from build123d import *

# Parameters (mm, degrees)
SKETCH1_W           = 4.7625
SKETCH1_H           = 101.6
BOSS_EXTRUDE1_DEPTH = 34.925
SKETCH2_W           = 101.6
SKETCH2_H           = 3.175
BOSS_EXTRUDE2_DEPTH = 152.4
SKETCH2_4_W         = 1.5875
SKETCH2_4_H         = 3.175
BOSS_EXTRUDE3_DEPTH = 25.4


with BuildPart() as part:
    # Sketch1 → Boss-Extrude1 (new body)
    with BuildSketch(Plane(origin=(0, -30.757642186, 0), x_dir=(-1, 0, 0), z_dir=(0, -1, 0))):
        with Locations((-83.04427371, -7.755970668)):
            Rectangle(SKETCH1_W, SKETCH1_H)
    extrude(amount=-BOSS_EXTRUDE1_DEPTH)

    # Sketch2 → Boss-Extrude2 (add)
    with BuildSketch(Plane.ZY.offset(-80.66302371)):
        with Locations((7.755970668, 2.579857814)):
            Rectangle(SKETCH2_W, SKETCH2_H)
    extrude(amount=BOSS_EXTRUDE2_DEPTH)

    # Sketch2<4> → Boss-Extrude3 (add)
    with BuildSketch(Plane.ZY.offset(-80.66302371)):
        with Locations((-39.075279332, -5.357642186)):
            Rectangle(SKETCH2_4_W, SKETCH2_4_H)
        with Locations((54.587220668, -5.357642186)):
            Rectangle(SKETCH2_4_W, SKETCH2_4_H)
    extrude(amount=BOSS_EXTRUDE3_DEPTH)


solid = part.part
Geometry: final body of the model. Coordinates: model frame, mm. A direction names the side the tool comes from. Coordinates: 2 decimals unless noted, no trailing zeros. Order: outer loops, then holes, each group sorted by start corner. A loop starts at its lowest first (then second) coordinate and runs counter-clockwise, first axis right, second up.
1) Set-up query: faces 4 (the flat face through (68, -5, -39.869)), 5 (the flat face through (68, -5, 53.793)), 6 (the flat face through (-71.737, 3, 7)), 7 (the flat face through (68, -5, 55.381)). Return all of +Z, -Z, +X, -X, +Y, -Y with unobstructed straight access to the full face (end or side cutting, diameter ignored); none if empty.
Result sheet:
face 4: -Z, -X, -Y
face 5: -X, -Y
face 6: +Z, -Z, -X, +Y, -Y
face 7: +Z, -X, -Y
2) Section C-C (y = -9). Return loops of the section in (x, z), then the cut area to 3 significant figures.
Result sheet:
outline: (80.66, -43.04) - (85.43, -43.04) - (85.43, 58.56) - (80.66, 58.56) - close
area: 484 mm2
3) Section D-D (x = 44). Return loops of the section in (y, z).
Result sheet:
outline: (0.99, -43.04) - (4.17, -43.04) - (4.17, 58.56) - (0.99, 58.56) - close
4) Draft query along Z for faces 1 (the flat face through (68, -5, -38.282)), 2 (the flat face through (6, 0.992, 7)), 3 (the flat face through (30, 2, 58.556)). Return one class per face: released by +Z, released by -Z, zero draft, split by the parting line, or undercut.
Result sheet:
face 1: undercut
face 2: zero draft
face 3: released by +Z
5) Section B-B (z = 30.5). Return loops of the section in (x, y), then the cut area to 3 significant figures.
Result sheet:
outline: (-71.74, 0.99) - (80.66, 0.99) - (80.66, -30.76) - (85.43, -30.76) - (85.43, 4.17) - (-71.74, 4.17) - close
area: 650 mm2
6) First-contact query: P1, Ø8, axis at y = -10.5, z = -12.5, coming from the -X side; P2, Ø3.5, axis at x = 70, y = -6, coming from the +Z side; P3, Ø8, axis at x = 36, z = -8, coming from the -Y side. Flat tips, straight axial feed; report the tip coordinate or a pass-through.
Result sheet:
P1: stops at x = 80.66
P2: stops at z = 55.38
P3: stops at y = 0.99
7) Section A-A (x = 74). Return loops of the section in (y, z), then the cut area to 3 significant figures.
Result sheet:
outline: (-6.95, -39.87) - (-3.77, -39.87) - (-3.77, -38.28) - (-6.95, -38.28) - close; (-6.95, 53.79) - (-3.77, 53.79) - (-3.77, 55.38) - (-6.95, 55.38) - close; (0.99, -43.04) - (4.17, -43.04) - (4.17, 58.56) - (0.99, 58.56) - close
area: 333 mm2
8) Ray query, probe 1 along X at (y, z) = (-8, -21); probe 2 along Y at (x, z) = (-48, -10). Return the intervals inside material, ascending.
Result sheet:
probe 1: x = 80.66 to 85.43
probe 2: y = 0.99 to 4.17
